Input: part model. Units: mm. Frame: model coordinates. A direction names the side the tool comes from. Coordinates: 2 decimals unless noted, no trailing zeros. Loops run counter-clockwise (first coordinate to the right, second up) from the corner with the lowest first, then second, coordinate; pieces in that order, holes last. Notation, with made-up numbers: (27.25, 65.25) -> (36.25, 65.25) arc R30 cw to (36.25, 89.25) -> close; hole circle Ø4 at (-39.75, 86). An arc over 180 degrees is marked (long way). Answer as a JSON object with one key per item and string values.
from build123d import *

# Parameters (mm, degrees)
BOSS_EXTRUDE1_DEPTH  = 20
FILLET1_R            = 2
M3_CLEARANCE_HOLE1_D = 3.4
SKETCH6_R            = 6.05
CUT_EXTRUDE1_DEPTH   = 39.1
M4_CLEARANCE_HOLE1_D = 4.5


with BuildPart() as part:
    # Sketch1 → Boss-Extrude1 (new body, symmetric)
    with BuildSketch(Plane.XY):
        Polygon((0, 0), (0, 50.8), (3.175, 50.8), (3.175, 3.175), (38.1, 3.175), (38.1, 0), align=None)
    extrude(amount=BOSS_EXTRUDE1_DEPTH, both=True)

    # Fillet1
    fillet1_edges = [part.edges().sort_by_distance(p)[0] for p in [
        (3.175, 3.175, 0),
    ]]
    fillet(fillet1_edges, radius=FILLET1_R)

    # M3 Clearance Hole1 (through all)
    with Locations(Plane.ZY):
        with Locations((0, 41.847738991), (13.553804618, 34.328139243), (-13.289066718, 18.830400251), (0, 10.852261009), (-13.289066718, 33.869599749), (13.553804618, 18.371860757)):
            Hole(M3_CLEARANCE_HOLE1_D / 2)

    # Sketch6 → Cut-Extrude1 (cut, through all)
    with BuildSketch(Plane.ZY):
        with Locations((7, 26.35)):
            Circle(SKETCH6_R)
    extrude(amount=-CUT_EXTRUDE1_DEPTH, mode=Mode.SUBTRACT)

    # M4 Clearance Hole1 (through all)
    with Locations(Plane(origin=(0, 3.175, 0), x_dir=(1, 0, 0), z_dir=(0, 1, 0))):
        with Locations((13.1, -12.5), (28.1, -12.5), (28.1, 12.5), (13.1, 12.5)):
            Hole(M4_CLEARANCE_HOLE1_D / 2)


solid = part.part
1. Mould query, pull axis Z, two halves, no side actions, for faces 3 (the face through (2, 50.8, 0)), 4 (the face through (2, 14, 20)), 5 (the face through (25.954, 1.565, -13.176)). Classes: pulls with the +Z half, pulls with the -Z half, needs draft (parallel to the pull), parting line crosses it, or undercut.
Reply:
{"face 3": "needs draft", "face 4": "pulls with the +Z half", "face 5": "undercut"}
2. Pin query (flat end, axial travel): P1, Ø5, axis at x = 10, z = -6.5, coming from the +Y side (3 decimals); P2, Ø20, axis at y = 25.5, z = 3, coming from the +X side (3 decimals). Return the tip coordinate at first contact, or that it passes through.
Reply:
{"P1": "stops at y = 3.175", "P2": "stops at x = 3.175"}
3. Section query B-B (y = 26.35). Return loops of the section in (x, z) (3 decimals), plus the area to 3 significant figures.
Reply:
{"outline": "(0, -20) -> (3.175, -20) -> (3.175, 0.95) -> (0, 0.95) -> close; (0, 13.05) -> (3.175, 13.05) -> (3.175, 20) -> (0, 20) -> close", "area": "88.6 mm2"}
4. Access query for faces 1 (the face through (21, 3.175, 0)), 2 (the face through (2, 14, -20)). Directions: +Z, -Z, +X, -X, +Y, -Y. A direction counts if a zero-diameter tool reaches every point of the face in a straight line with its end or side. Return the directions, or none.
Reply:
{"face 1": "+Z, -Z, +X, +Y", "face 2": "-Z, +X, -X, +Y, -Y"}
5. Section query D-D (z = -13.5). Return loops of the section in (x, y) (3 decimals), plus the area to 3 significant figures.
Reply:
{"outline": "(0, 0) -> (11.084, 0) -> (11.084, 3.175) -> (5.175, 3.175) arc R2 cw to (3.175, 5.175) -> (3.175, 17.144) -> (0, 17.144) -> close; (0, 20.517) -> (3.175, 20.517) -> (3.175, 32.183) -> (0, 32.183) -> close; (0, 35.556) -> (3.175, 35.556) -> (3.175, 50.8) -> (0, 50.8) -> close; (15.116, 0) -> (26.084, 0) -> (26.084, 3.175) -> (15.116, 3.175) -> close; (30.116, 0) -> (38.1, 0) -> (38.1, 3.175) -> (30.116, 3.175) -> close", "area": "226 mm2"}
6. Section query A-A (z = 0). Return loops of the section in (x, y) (3 decimals), plus the area to 3 significant figures.
Reply:
{"outline": "(0, 0) -> (38.1, 0) -> (38.1, 3.175) -> (5.175, 3.175) arc R2 cw to (3.175, 5.175) -> (3.175, 9.152) -> (0, 9.152) -> close; (0, 12.552) -> (3.175, 12.552) -> (3.175, 40.148) -> (0, 40.148) -> close; (0, 43.548) -> (3.175, 43.548) -> (3.175, 50.8) -> (0, 50.8) -> close", "area": "251 mm2"}
7. Line query: line 1 along Z through (x, y) = (28, 1); line 2 along X through (y, z) = (2.1, -12.5); line 3 along Y through (x, z) = (1.55, 0). Output: solid intervals per line, ascending.
Reply:
{"line 1": "z = -20 to -14.75, -10.25 to 10.25, 14.75 to 20", "line 2": "x = 0 to 10.85, 15.35 to 25.85, 30.35 to 38.1", "line 3": "y = 0 to 9.15, 12.55 to 40.15, 43.55 to 50.8"}
8. Section query C-C (x = 28.1). Return loops of the section in (y, z) (3 decimals).
Reply:
{"outline": "(0, -20) -> (3.175, -20) -> (3.175, -14.75) -> (0, -14.75) -> close; (0, -10.25) -> (3.175, -10.25) -> (3.175, 10.25) -> (0, 10.25) -> close; (0, 14.75) -> (3.175, 14.75) -> (3.175, 20) -> (0, 20) -> close"}
